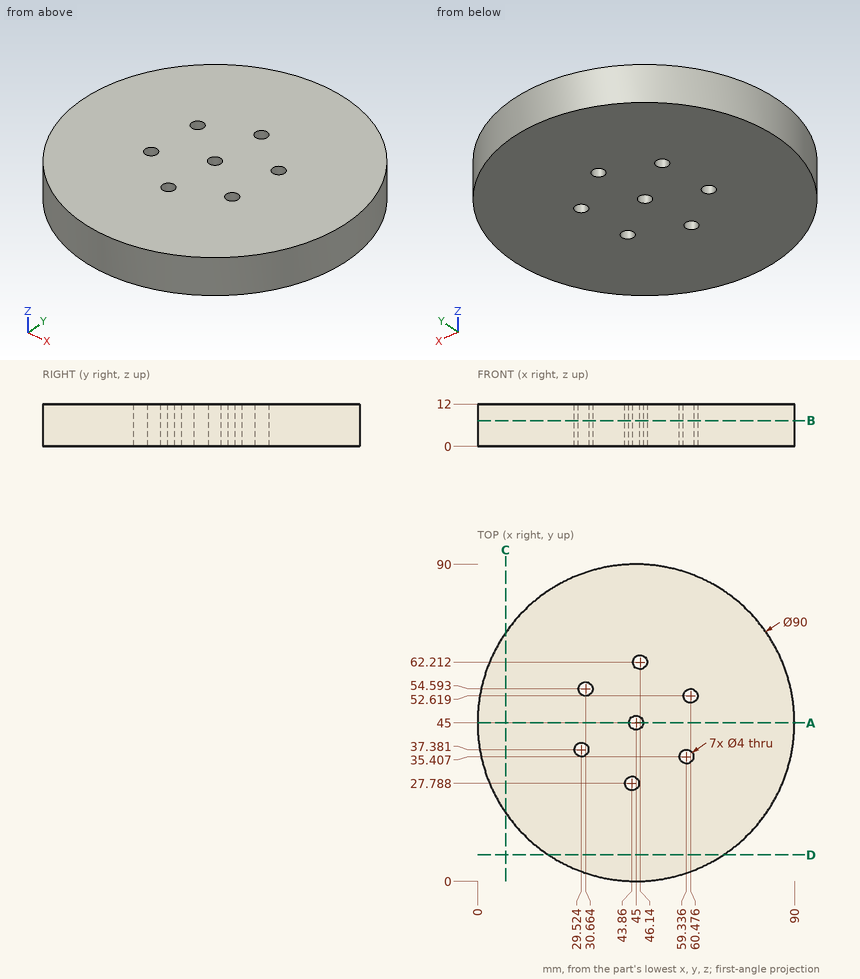
Input: dimensioned drawing with shaded views. Units: mm. Origin: part minimum x, y, z. Round coordinates to 2 decimals unless told otherwise and drop trailing zeros. Order: outer loops, then holes, each group sorted by start corner. A loop starts at its lowest first (then second) coordinate and runs counter-clockwise, first axis right, second up. Notation, with made-up numbers: (-7.5, 75.25) - (28.5, 75.25) arc R21 ccw to (28.5, 81.25) - close; hole circle Ø8 at (44, 86.5). An arc over 180 degrees is marked (long way). Use CSV: the item, a comma, the result in double quotes. Start each with the question number.
Q1. Section query D-D (y = 7.5). Return loops of the section in (x, z) (1 decimal).
Q2. Section query B-B (z = 7.25). Return loops of the section in (x, y).
Q3. First-contact query: pin 1 (3.5 mm diameter, centred on x = 30.66, y = 54.59, fed in from +Z) (3 decimals); pin 2 (5 mm diameter, centred on y = 38.5, z = 4.5, fed in from -X); pin 3 (1 mm diameter, centred on y = 19, z = 5, fed in from +X); pin 4 (3 mm diameter, centred on x = 23, z = 8, fed in from -Y). Flat tips, straight axial feed; report the tip coordinate or a pass-through.
Q4. Section query A-A (y = 45). Return loops of the section in (x, z), and give its area (3 significant figures).
Q5. Section query C-C (x = 8). Return loops of the section in (y, z), and give its area (3 significant figures).
Q6. Material intervals for line 1 along Y through (x, z) = (45, 9) (1 decimal); line 2 along X through (y, z) = (53, 6.75) (1 decimal); line 3 along X through (y, z) = (46.5, 5.75) (1 decimal), sorted ascending. Write a range as from..to.
Result set:
1,outline,"(20.1, 0) - (69.9, 0) - (69.9, 12) - (20.1, 12) - close"
2,outline,"circle Ø90 at (45, 45); hole circle Ø4 at (29.52, 37.38); hole circle Ø4 at (30.66, 54.59); hole circle Ø4 at (43.86, 27.79); hole circle Ø4 at (45, 45); hole circle Ø4 at (46.14, 62.21); hole circle Ø4 at (59.34, 35.41); hole circle Ø4 at (60.48, 52.62)"
3,pin 1,"passes through"
3,pin 2,"stops at x = 0.18"
3,pin 3,"stops at x = 82.08"
3,pin 4,"stops at y = 4.94"
4,outline,"(0, 0) - (43, 0) - (43, 12) - (0, 12) - close; (47, 0) - (90, 0) - (90, 12) - (47, 12) - close"
4,area,"1,030 mm2"
5,outline,"(19.39, 0) - (70.61, 0) - (70.61, 12) - (19.39, 12) - close"
5,area,"615 mm2"
6,line 1,"y = 0..26.1, 29.4..43, 47..60.6, 63.9..90"
6,line 2,"x = 0.7..29.5, 31.9..58.5, 62.4..89.3"
6,line 3,"x = 0..43.7, 46.3..90"
